Here's how the part is built. I have some questions about the finished solid (model axes, mm). A direction names the side the tool comes from. Coordinates: 2 decimals unless noted, no trailing zeros. Loops run counter-clockwise (first coordinate to the right, second up) from the corner with the lowest first, then second, coordinate; pieces in that order, holes last. Notation, with made-up numbers: (-19, 53) -> (0, 53) arc R26 cw to (0, 86) -> close; hole circle Ø3 at (-36, 31.25). An arc over 180 degrees is marked (long way). Answer as a JSON object with one key per item and string values. Group by question number.
1) If we mould it in two halves opening along Y, with no side actions, what happens to faces 1 (the flat face through (-8, 47, 0.7)), 2 (the flat face through (48.2, -43.4, 6.3)), 3 (the cylindrical face through (60.967, -25.278, 4.38))? For each: +Y half, -Y half, draft (parallel to the pull), parting line (faces both ways), or undercut.
2) I want a section at A-A (z = 2). Write out the boundary of the cut face in (x, y), then the cut area to 3 significant figures.
3) I need wall thicknesses on probe 1 along Y at (x, z) = (7.8, 1.55); probe 2 along X at (y, z) = (7.8, 1.9); probe 3 along Y at (x, z) = (26, 1.5). Which ranges of each line are inside material? Lowest first, please. Write a range as [from, to].
4) Which directions (+Z, -Z, +X, -X, +Y, -Y) give clear straight access to the entire face, cutting with the end or side of a thin tool? Please do faces 4 (the flat face through (32, 1, 0)), 5 (the flat face through (8, -47, 0.7)).
5) I'm going to push flat-ended pins straight in: pin 1 (1.5 mm diameter, centred on x = 21.5, z = 4, fed in from -Y); pin 2 (4.5 mm diameter, centred on x = 48, y = 8.5, fed in from +Z); pin 3 (3 mm diameter, centred on x = 63.9, y = 59.6, fed in from +Z); pin 4 (1.2 mm diameter, centred on x = -7.5, y = 47, fed in from +Z). Where does each tip first touch, or does it pass through?
```python
from build123d import *

# Parameters (mm, degrees)
F0_W     = 150
F0_H     = 150
F0_W_2   = 60
F0_H_2   = 60
F1_DEPTH = 3
F2_R     = 66
F2_R_2   = 64
F3_DEPTH = 3.3
F5_DEPTH = 2.3
F6_R     = 0.5
F7_R     = 0.5
F4_R     = 1.75
F8_DEPTH = 25


# Not quite as in the source:
# - a feature names something its author has since deleted; it is built from what else it names


with BuildPart() as f1:
    # F0 (on Top) → F1 (new body)
    with BuildSketch(Plane.XY):
        Rectangle(F0_W, F0_H)
        Rectangle(F0_W_2, F0_H_2, mode=Mode.SUBTRACT)
    extrude(amount=F1_DEPTH)

    # F2 (on face) → F3 (join)
    with BuildSketch(Plane.XY.offset(3)):
        Circle(F2_R)
        Circle(F2_R_2, mode=Mode.SUBTRACT)
    extrude(amount=F3_DEPTH)

    # F4 (on face) → F5 (cut)
    with BuildSketch(Plane.XY.offset(3)):
        with BuildLine():
            ThreePointArc((-49.1, -7.8), (-48.5142135624, -9.2142135624), (-47.1, -9.8))
            Line((-47.1, -9.8), (-47.1, -7.8))
            Line((-47.1, -7.8), (-49.1, -7.8))
        make_face()
        with BuildLine():
            Line((-47.1, -7.8), (-47.1, -9.8))
            ThreePointArc((-47.1, -9.8), (-45.6857864376, -9.2142135624), (-45.1, -7.8))
            ThreePointArc((-45.1, -7.8), (-47.1, -5.8), (-49.1, -7.8))
            Line((-49.1, -7.8), (-47.1, -7.8))
        make_face()
        with BuildLine():
            Line((-7.8, 47.2), (-9.8, 47.2))
            ThreePointArc((-9.8, 47.2), (-7.8, 45.2), (-5.8, 47.2))
            ThreePointArc((-5.8, 47.2), (-6.3857864376, 48.6142135624), (-7.8, 49.2))
            Line((-7.8, 49.2), (-7.8, 47.2))
        make_face()
        with BuildLine():
            ThreePointArc((-7.8, 49.2), (-9.2142135624, 48.6142135624), (-9.8, 47.2))
            Line((-9.8, 47.2), (-7.8, 47.2))
            Line((-7.8, 47.2), (-7.8, 49.2))
        make_face()
        with BuildLine():
            Line((47.1, 7.8), (47.1, 9.8))
            ThreePointArc((47.1, 9.8), (45.6857864376, 6.3857864376), (49.1, 7.8))
            Line((49.1, 7.8), (47.1, 7.8))
        make_face()
        with BuildLine():
            ThreePointArc((49.1, 7.8), (48.5142135624, 9.2142135624), (47.1, 9.8))
            Line((47.1, 9.8), (47.1, 7.8))
            Line((47.1, 7.8), (49.1, 7.8))
        make_face()
        with BuildLine():
            ThreePointArc((9.8, -47.1), (6.3857864376, -45.6857864376), (7.8, -49.1))
            Line((7.8, -49.1), (7.8, -47.1))
            Line((7.8, -47.1), (9.8, -47.1))
        make_face()
        with BuildLine():
            Line((7.8, -47.1), (7.8, -49.1))
            ThreePointArc((7.8, -49.1), (9.2142135624, -48.5142135624), (9.8, -47.1))
            Line((9.8, -47.1), (7.8, -47.1))
        make_face()
    extrude(amount=-F5_DEPTH, mode=Mode.SUBTRACT)

    # F6
    f6_edges = [f1.edges().sort_by_distance(p)[0] for p in [
        (-66, 0, 6.3),
    ]]
    fillet(f6_edges, radius=F6_R)

    # F7
    f7_edges = [f1.edges().sort_by_distance(p)[0] for p in [
        (-64, 0, 6.3),
    ]]
    fillet(f7_edges, radius=F7_R)

    # F4 (on face) → F8 (cut)
    with BuildSketch(Plane.XY.offset(3)):
        with Locations((63.9, 59.6)):
            Circle(F4_R)
    extrude(amount=-F8_DEPTH, mode=Mode.SUBTRACT)


solid = f1.part
```
Determined:
{
 "1": {"face 1": "undercut", "face 2": "draft", "face 3": "parting line"},
 "2": {"outline": "(-75, -75) -> (75, -75) -> (75, 75) -> (-75, 75) -> close; hole circle Ø4 at (-47.1, -7.8); hole (-30, -30) -> (30, -30) -> (30, 30) -> (-30, 30) -> close; hole circle Ø4 at (-7.8, 47.2); hole circle Ø4 at (7.8, -47.1); hole circle Ø4 at (47.1, 7.8); hole circle Ø3.5 at (63.9, 59.6)", "area": "18,800 mm^2"},
 "3": {"probe 1": "[-75, -49.1], [-45.1, -30], [30, 75]", "probe 2": "[-75, -30], [30, 45.1], [49.1, 75]", "probe 3": "[-75, -30], [30, 75]"},
 "4": {"face 4": "-Z, +X, -X, +Y, -Y", "face 5": "+Z"},
 "5": {"pin 1": "y = -62.65", "pin 2": "z = 3", "pin 3": "through", "pin 4": "z = 0.7"}
}
